Work out the finished part from the listing and answer in its coordinate system (mm). A direction names the side the tool comes from. Give positions to 0.01 mm unless a question says otherwise; leave off trailing zeros. Loops run counter-clockwise (first coordinate to the right, second up) from the corner with the lowest first, then second, coordinate; pieces in that order, holes last. Notation, with made-up numbers: (35, 75) - (57, 75) arc R14 cw to (57, 97) - close; hole circle Ø4 at (11, 78). An arc over 180 degrees is marked (long way). One line per item, written item: value.
from build123d import *
from build123d import SkipClean  # not in build123d's __all__

# Parameters (mm, degrees)
F0_R      = 2.5
F1_DEPTH  = 36.5
F3_START  = 9.5
F2_R      = 3.25
F3_DEPTH  = 10
F5_DEPTH  = 3
F7_START  = -6.8
F7_DEPTH  = 18.2
F8_R      = 2
F9_DEPTH  = 3.501
F10_R     = 2.99999
F12_DEPTH = 2.5
F13_SIZE  = 0.9999
F14_R     = 2
F15_DEPTH = 2


# Not quite as in the source:
# - a fillet or chamfer is up to 0.001 mm smaller than in the source, because OpenCascade refuses the exact size
# - after a boolean that leaves OpenCascade's solid faulty, fix() repairs it
# - ends of sketch curves that miss each other by under 0.0002 mm in the source are joined


with BuildPart() as f1:
    # F0 (on Top) → F1 (new body)
    with BuildSketch(Plane.XY):
        Circle(F0_R)
    extrude(amount=F1_DEPTH)

    # F2 (on Top) → F3 (join)
    with BuildSketch(Plane.XY.offset(F3_START)):
        Circle(F2_R)
    extrude(amount=F3_DEPTH)

    # F4 (on Right) → F5 (join, symmetric)
    with BuildSketch(Plane.YZ):
        with BuildLine():
            Line((0, 13), (0, 9.5))
            Line((0, 9.5), (6.25, 9.5))
            ThreePointArc((6.25, 9.5), (6.9571067812, 9.2071067812), (7.25, 8.5))
            Line((7.25, 8.5), (7.25, 0))
            ThreePointArc((7.25, 0), (8.5680194847, -3.1819805153), (11.75, -4.5))
            Line((11.75, -4.5), (27.25, -4.5))
            Line((27.25, -4.5), (27.25, -1))
            Line((27.25, -1), (11.75, -1))
            ThreePointArc((11.75, -1), (11.0428932188, -0.7071067812), (10.75, 0))
            Line((10.75, 0), (10.75, 8.5))
            ThreePointArc((10.75, 8.5), (9.4319805153, 11.6819805153), (6.25, 13))
            Line((6.25, 13), (0, 13))
        make_face()
    extrude(amount=F5_DEPTH, both=True)

    # F6 (on face) → F7 (join)
    with BuildSketch(Plane.XY.offset(36.5).offset(F7_START)):
        with BuildLine():
            ThreePointArc((3.0434027778, -1.1402629224), (3, 0), (3.0434027778, 1.1402629224))
            ThreePointArc((3.0434027778, 1.1402629224), (2.8145825623, 1.625), (2.5091980467, 2.0655326583))
            ThreePointArc((2.5091980467, 2.0655326583), (1.5, 2.5980762114), (0.5342047311, 3.2057955807))
            ThreePointArc((0.5342047311, 3.2057955807), (0, 3.25), (-0.5342047311, 3.2057955807))
            ThreePointArc((-0.5342047311, 3.2057955807), (-1.5, 2.5980762114), (-2.5091980467, 2.0655326583))
            ThreePointArc((-2.5091980467, 2.0655326583), (-2.8145825623, 1.625), (-3.0434027778, 1.1402629224))
            ThreePointArc((-3.0434027778, 1.1402629224), (-3, 0), (-3.0434027778, -1.1402629224))
            ThreePointArc((-3.0434027778, -1.1402629224), (-2.8145825623, -1.625), (-2.5091980467, -2.0655326583))
            ThreePointArc((-2.5091980467, -2.0655326583), (-1.5, -2.5980762114), (-0.5342047311, -3.2057955807))
            ThreePointArc((-0.5342047311, -3.2057955807), (0, -3.25), (0.5342047311, -3.2057955807))
            ThreePointArc((0.5342047311, -3.2057955807), (1.5, -2.5980762114), (2.5091980467, -2.0655326583))
            ThreePointArc((2.5091980467, -2.0655326583), (2.8145825623, -1.625), (3.0434027778, -1.1402629224))
        make_face()
    with SkipClean():  # cleaning this boolean's faces spoils the solid; the shape is the same uncleaned
        extrude(amount=-F7_DEPTH)

    # F8 (on face) → F9 (cut, through all)
    with BuildSketch(Plane.XY.offset(-1)):
        with Locations((0, 24.25)):
            Circle(F8_R)
    extrude(amount=-F9_DEPTH, mode=Mode.SUBTRACT)

    add(f1.part.fix(), mode=Mode.REPLACE)

    # F10 (radius 3 in the source; OpenCascade refuses exactly that, so slightly less here)
    f10_edges = [f1.edges().sort_by_distance(p)[0] for p in [
        (-3, 27.25, -2.75),
        (3, 27.25, -2.75),
    ]]
    fillet(f10_edges, radius=F10_R)

    # F11 (on face) → F12 (cut)
    with BuildSketch(Plane(origin=(0, 0, 0), x_dir=(1, 0, 0), z_dir=(0, 0, -1))):
        with BuildLine():
            ThreePointArc((1.6903389552, -1.8419430546), (2.1650635095, -1.25), (2.4403389552, -0.5429049489))
            Line((2.4403389552, -0.5429049489), (-1.6903389552, 1.8419430546))
            ThreePointArc((-1.6903389552, 1.8419430546), (-2.1650635095, 1.25), (-2.4403389552, 0.5429049489))
            Line((-2.4403389552, 0.5429049489), (1.6903389552, -1.8419430546))
        make_face()
    extrude(amount=-F12_DEPTH, mode=Mode.SUBTRACT)

    # F13 (size 1 in the source; OpenCascade refuses exactly that, so slightly less here)
    f13_edges = [f1.edges().sort_by_distance(p)[0] for p in [
        (-1.25, 2.165064, 0),
        (-2.5, 0, 36.5),
        (1.00602, -2.288651, 0),
    ]]
    chamfer(f13_edges, length=F13_SIZE)

    # F14 (on face) → F15 (join)
    with BuildSketch(Plane.XY.offset(-1)):
        with BuildLine():
            Line((3, 24.25), (3, 15.5))
            Line((3, 15.5), (4, 16.5))
            Line((4, 16.5), (4, 24.25))
            ThreePointArc((4, 24.25), (3.1213203436, 26.3713203436), (1, 27.25))
            Line((1, 27.25), (0, 27.25))
            ThreePointArc((0, 27.25), (2.1213203436, 26.3713203436), (3, 24.25))
        make_face()
        with BuildLine():
            Line((3, 11.75), (3, 15.5))
            Line((3, 15.5), (3, 24.25))
            ThreePointArc((3, 24.25), (2.1213203436, 26.3713203436), (0, 27.25))
            ThreePointArc((0, 27.25), (-2.1213232725, 26.3713232725), (-3, 24.25001))
            Line((-3, 24.25001), (-3, 11.75))
            Line((-3, 11.75), (3, 11.75))
        make_face()
        with Locations((0, 24.25)):
            Circle(F14_R, mode=Mode.SUBTRACT)
    extrude(amount=-F15_DEPTH)


solid = f1.part
1. Section D-D (y = 8) is taken. Write down the section's boundary in (x, z), and give its area (3 significant figures).
Output:
outline: (-3, -2.49) - (3, -2.49) - (3, 12.65) - (-3, 12.65) - close
area: 90.8 mm²
2. For faces 4 (the flat face through (3.3, 21.8, -3)), 5 (the flat face through (0, 7.25, 4)), 6 (the flat face through (0.404, -0.633, 1.232)), determine the directions among +Z, -Z, +X, -X, +Y, -Y from which every point of the face is accessible in a straight line to the end or side of a thin tool.
Output:
face 4: -Z, +X, +Y
face 5: -Z, +X, -X
face 6: -Z
3. Find the intervals of material crossed by line 1 along X through (y, z) = (24, -4); line 2 along Z through (x, y) = (-2, 20.5); line 3 along Y through (x, z) = (0, -3.85), in increasing order.
Output:
line 1: x = -3 to -1.98, 1.98 to 3
line 2: z = -4.5 to -1
line 3: y = 9.42 to 22.25, 26.25 to 27.25
4. Section B-B (y = 17) is taken. Write down the section's boundary in (x, z), and give its area (3 significant figures).
Output:
outline: (-3, -4.5) - (3, -4.5) - (3, -3) - (4, -3) - (4, -1) - (-3, -1) - close
area: 23.0 mm²
5. Flat-ended cylindrical pins translate along their axes: pin 1 Ø10 at (y, z) = (7.5, 2) entering from -X; pin 2 Ø1.3 at (x, y) = (1, -2.5) entering from +Z; pin 3 Ø0.8 at (x, y) = (0, -1) entering from -Z. Find the tip coordinate at first contact, or state that the pin passes through.
Output:
pin 1: stops at x = -3
pin 2: stops at z = 35.96
pin 3: stops at z = 0
6. Section A-A (z = 29) is taken. Write down the section's boundary in (x, y), and give its area (3 significant figures).
Output:
outline: (-3.04, -1.14) arc R3.25 ccw to (-2.51, -2.07) arc R15 cw to (-0.53, -3.21) arc R3.25 ccw to (0.53, -3.21) arc R15 cw to (2.51, -2.07) arc R3.25 ccw to (3.04, -1.14) arc R15 cw to (3.04, 1.14) arc R3.25 ccw to (2.51, 2.07) arc R15 cw to (0.53, 3.21) arc R3.25 ccw to (-0.53, 3.21) arc R15 cw to (-2.51, 2.07) arc R3.25 ccw to (-3.04, 1.14) arc R15 cw to start
area: 30.9 mm²
7. Section C-C (z = 17) is taken. Write down the section's boundary in (x, y), and give its area (3 significant figures).
Output:
outline: circle Ø6.5 at (0, 0)
area: 33.2 mm²
8. The mould has two halves that part along Y. Classify faces 1 (the flat face through (0, 20, -1)), 2 (the cylindrical face through (-0.54, -2.44, 32.56)), 3 (the flat face through (0, 0, 2.5)): released by +Y, released by -Y, zero draft, split by the parting line, or undercut.
Output:
face 1: zero draft
face 2: split by the parting line
face 3: undercut
